Can you work these out from the model? Positions are in its coordinate system, mm. A direction names the side the tool comes from. Round coordinates to 2 decimals unless told otherwise and drop trailing zeros. Loops run counter-clockwise (first coordinate to the right, second up) from the corner with the lowest first, then second, coordinate; pieces in that order, holes last. Notation, with made-up numbers: M 25.25,-35.75 L 56.25,-35.75 A6 ccw 56.25,-25.75 Z; hole C 34.5,-4 d3. An arc over 180 degrees is marked long. Answer as CSV lines item,"result".
from build123d import *

# Parameters (mm, degrees)
F0_W     = 501.1803507805
F0_H     = 32.8778875992
F1_DEPTH = 1000


with BuildPart() as f1:
    # F0 (on Top) → F1 (new body)
    with BuildSketch(Plane.XY):
        Polygon((-352.7414500713, 0.8144499734), (-352.7414500713, 33.6923375726), (-383.2314908504, 33.6923375726), (-383.2314908504, -166.3986742496), (-352.7414500713, -166.3986742496), align=None)
        with Locations((-102.1512746811, 17.253393773)):
            Rectangle(F0_W, F0_H)
        Polygon((177.9761463404, 33.6923375726), (148.4389007092, 33.6923375726), (148.4389007092, 0.8144499734), (148.4389007092, -166.3986742496), (177.9761463404, -166.3986742496), align=None)
    extrude(amount=F1_DEPTH)


solid = f1.part
Item 1: Will this pin go through, and if not, where does the flat tip stop? pin 1 (3 mm diameter, centred on x = -55, z = 199, fed in from -Y).
Output:
pin 1,"stops at y = 0.81"
Item 2: If we section it at C-C on x = -23.5: Write out the boundary of the cut face in (y, z), then the cut area to 3 significant figures.
Output:
outline,"M 0.81,0 L 33.69,0 L 33.69,1000 L 0.81,1000 Z"
area,"32,900 mm2"
Item 3: If we section it at B-B on z = 684: Write out the boundary of the cut face in (x, y), then the cut area to 3 significant figures.
Output:
outline,"M -383.23,-166.4 L -352.74,-166.4 L -352.74,0.81 L 148.44,0.81 L 148.44,-166.4 L 177.98,-166.4 L 177.98,33.69 L -383.23,33.69 Z"
area,"28,500 mm2"
Item 4: If I drill on line 1 along X through (y, z) = (-3, 63); line 2 along Y through (x, z) = (-35, 317.5), over which ranges is the centre line in solid material (lowest first)? Write a range as from..to.
Output:
line 1,"x = -383.23..-352.74, 148.44..177.98"
line 2,"y = 0.81..33.69"
Item 5: On a 3-axis mill with a long thin cutter (end or side, diameter ignored), from which of +Z, -Z, +X, -X, +Y, -Y can I reach the whole of each face in a straight line? I mean faces 5 (the face through (177.976, -68, 493)), 6 (the face through (148.439, -82, 493)). Say none if no direction works.
Output:
face 5,"+Z, -Z, +X, +Y, -Y"
face 6,"+Z, -Z, -Y"
Item 6: If we section it at A-A on y = -125: Write out the boundary of the cut face in (x, z), then the cut area to 3 significant figures.
Output:
outline,"M -383.23,0 L -352.74,0 L -352.74,1000 L -383.23,1000 Z; M 148.44,0 L 177.98,0 L 177.98,1000 L 148.44,1000 Z"
area,"60,000 mm2"
Item 7: We'd pull the mould along X, two halves only. Please class faces 1 (the face through (-352.741, -84, 493)), 2 (the face through (-383.231, -65, 493)), 3 (the face through (-368, -166.399, 493)), 4 (the face through (-106, 0.814, 493)): released by +X, released by -X, zero draft, split by the parting line, or undercut.
Output:
face 1,"undercut"
face 2,"released by -X"
face 3,"zero draft"
face 4,"undercut"
